from build123d import *

# Parameters (mm, degrees)
F1_DEPTH  = 20
F3_DEPTH  = 10
F4_R      = 1.25
F5_DEPTH  = 2.2
F7_DEPTH  = 10
F9_R      = 1.25
F10_DEPTH = 28.001
F11_R     = 2
F14_DEPTH = 1.5
F16_W     = 20
F16_H     = 10
F17_DEPTH = 26.7
F19_R     = 1.25
F20_DEPTH = 32.1
F22_W     = 20
F22_H     = 9.2705127583
F23_DEPTH = 6.9
F24_DEPTH = 2.9
F25_R     = 1.25
F26_DEPTH = 12.5


with BuildPart() as f1:
    # F0 (on Top) → F1 (new body)
    with BuildSketch(Plane.XY):
        with BuildLine():
            Line((-17.4218026286, 7.8075558554), (-19.6106751933, 7.8075558554))
            ThreePointArc((-19.6106751933, 7.8075558554), (-13.947676921, -0.1749805422), (-8.2846786486, 7.8075558554))
            Line((-8.2846786486, 7.8075558554), (-10.4735512133, 7.8075558554))
            ThreePointArc((-10.4735512133, 7.8075558554), (-13.947676921, 1.8250194578), (-17.4218026286, 7.8075558554))
        make_face()
    extrude(amount=F1_DEPTH)

    # F2 (on Top) → F3 (join, symmetric)
    with BuildSketch(Plane.XY):
        Polygon((-3.947676921, 1.8250194578), (-13.947676921, 1.8250194578), (-23.947676921, 1.8250194578), (-23.947676921, -1.1749805422), (-3.947676921, -1.1749805422), align=None)
    extrude(amount=F3_DEPTH, both=True)

    # F4 (on Front) → F5 (cut, symmetric)
    with BuildSketch(Plane.XZ):
        with Locations((-9.197676921, -6)):
            Circle(F4_R)
        with Locations((-18.697676921, -6)):
            Circle(F4_R)
    extrude(amount=F5_DEPTH, both=True, mode=Mode.SUBTRACT)

    # F6 (on face) → F7 (join, through all)
    with BuildSketch(Plane.XY.offset(10)):
        with BuildLine():
            Line((-3.947676921, 1.8250194578), (-9.475540966, 1.8250194578))
            ThreePointArc((-9.475540966, 1.8250194578), (-13.947676921, -0.1749805422), (-18.419812876, 1.8250194578))
            Line((-18.419812876, 1.8250194578), (-23.947676921, 1.8250194578))
            Line((-23.947676921, 1.8250194578), (-23.947676921, -1.1749805422))
            Line((-23.947676921, -1.1749805422), (-3.947676921, -1.1749805422))
            Line((-3.947676921, -1.1749805422), (-3.947676921, 1.8250194578))
        make_face()
    extrude(amount=F7_DEPTH)

    # F9 (on offset) → F10 (cut, through all)
    with BuildSketch(Plane(origin=(0, 26.8250194578, 0), x_dir=(-1, 0, 0), z_dir=(0, 1, 0))):
        with Locations((23.947676921, -6)):
            Circle(F9_R)
        with Locations((3.947676921, -6)):
            Circle(F9_R)
    extrude(amount=-F10_DEPTH, mode=Mode.SUBTRACT)

    # F11
    f11_edges = [f1.edges().sort_by_distance(p)[0] for p in [
        (-23.947677, 0.325019, -10),
        (-3.947677, 0.325019, -10),
    ]]
    fillet(f11_edges, radius=F11_R)

    # F13 (on offset) → F14 (join)
    with BuildSketch(Plane.XZ.offset(1.1749805422)):
        with BuildLine():
            ThreePointArc((-23.947676921, -4.75), (-22.697676921, -6), (-23.947676921, -7.25))
            Line((-23.947676921, -7.25), (-23.947676921, -8))
            ThreePointArc((-23.947676921, -8), (-23.3618904833, -9.4142135624), (-21.947676921, -10))
            Line((-21.947676921, -10), (-5.947676921, -10))
            ThreePointArc((-5.947676921, -10), (-4.5334633586, -9.4142135624), (-3.947676921, -8))
            Line((-3.947676921, -8), (-3.947676921, -7.25))
            ThreePointArc((-3.947676921, -7.25), (-5.197676921, -6), (-3.947676921, -4.75))
            Line((-3.947676921, -4.75), (-3.947676921, 20))
            Line((-3.947676921, 20), (-23.947676921, 20))
            Line((-23.947676921, 20), (-23.947676921, -4.75))
        make_face()
    extrude(amount=F14_DEPTH)

    # F16 (on offset) → F17 (cut)
    with BuildSketch(Plane(origin=(0, 26.8250194578, 0), x_dir=(-1, 0, 0), z_dir=(0, 1, 0))):
        with Locations((13.947676921, -5)):
            Rectangle(F16_W, F16_H)
    extrude(amount=-F17_DEPTH, mode=Mode.SUBTRACT)

    # F19 (on offset) → F20 (cut)
    with BuildSketch(Plane.XZ.offset(25)):
        with Locations((-9.197676921, -6)):
            Circle(F19_R)
        with Locations((-18.697676921, -6)):
            Circle(F19_R)
    extrude(amount=-F20_DEPTH, mode=Mode.SUBTRACT)

    # F22 (on offset) → F23 (cut)
    with BuildSketch(Plane.XY.offset(11.9)):
        with Locations((-13.947676921, 6.460275837)):
            Rectangle(F22_W, F22_H)
    extrude(amount=-F23_DEPTH, mode=Mode.SUBTRACT)

    # F22 (on offset) → F24 (cut)
    with BuildSketch(Plane.XY.offset(11.9)):
        with Locations((-13.947676921, 6.460275837)):
            Rectangle(F22_W, F22_H)
    extrude(amount=F24_DEPTH, mode=Mode.SUBTRACT)

    # F25 (on offset) → F26 (cut, symmetric)
    with BuildSketch(Plane(origin=(0, 1.8250194578, 0), x_dir=(-1, 0, 0), z_dir=(0, 1, 0))):
        with Locations((8.2846786486, 10.0688289385)):
            Circle(F25_R)
        with Locations((19.6106751933, 10.0688289385)):
            Circle(F25_R)
    extrude(amount=F26_DEPTH, both=True, mode=Mode.SUBTRACT)


solid = f1.part
Geometry check sheet. Reference: the model listing, model coordinates, mm. A direction names the side the tool comes from. Give positions to 0.01 mm unless a question says otherwise; leave off trailing zeros. Write each loop counter-clockwise with the first axis right and the second up, starting at its lowest first coordinate (ties: lowest second). Pieces come first, ordered by that corner, then holes. Notation, with made-up numbers: M -15,-4 L 40,-4 A18 ccw 40,23 Z; hole C 71.5,-6.75 d10. An arc over 180 degrees is marked long. Answer as CSV lines item,"result". Start each with the question number.
Q1. Section check B-B, the plane y = 3.25. Record the cut outline in (x, z), then the cut area to 3 significant figures.
Q2. Go/stop test with flat-tipped pins: pin 1 (5 mm diameter, centred on x = -18, y = 3.5, fed in from -Z); pin 2 (3 mm diameter, centred on x = -8.28, z = 10.07, fed in from +Y) (3 decimals). Record where each tip stops, or that it passes through.
Q3. Release check for a two-part mould opening along X. For faces 1 (the face through (-22.7, -1.26, -5.97)), 2 (the face through (-14, -1, -10)), 3 (the face through (-8.01, -0.39, 8.85)), 4 (the face through (-13.831, 1.827, 2.465)) record: pulls with the +X half, pulls with the -X half, needs draft (parallel to the pull), parting line crosses it, or undercut.
Q4. Section check A-A, the plane z = -6. Record the cut outline in (x, y).
Q5. Material ranges on L1, parallel to Z at x = -9.5, y = 4.75; L2, parallel to Y at x = -7.25, z = 6; L3, parallel to Y at x = -15.75, z = -3.75, recorded low to high.
Q6. Section check C-C, the plane z = 17.75. Record the cut outline in (x, y).
Q7. Section check D-D, the plane x = -19.25. Record the cut outline in (y, z).
Q8. Tool access check on faces 5 (the face through (-9, 7.808, 17)), 6 (the face through (-14, 1, 0)), 7 (the face through (-18.3, 4.9, 5)). Record the directions out of +Z, -Z, +X, -X, +Y, -Y that give a thin tool (end or side, any length) a straight path to the whole face; none if there is none.
Geometry says:
1,outline,"M -19.37,0 L -17.01,0 L -17.01,5 L -19.37,5 Z; M -19.37,14.8 L -17.01,14.8 L -17.01,20 L -19.37,20 Z; M -10.89,0 L -8.53,0 L -8.53,5 L -10.89,5 Z; M -10.89,14.8 L -8.53,14.8 L -8.53,20 L -10.89,20 Z"
1,area,"48.1 mm^2"
2,pin 1,"z = 0"
2,pin 2,"y = 1.825"
3,face 1,"pulls with the -X half"
3,face 2,"needs draft"
3,face 3,"undercut"
3,face 4,"undercut"
4,outline,"M -22.7,-2.67 L -19.95,-2.67 L -19.95,0.13 L -22.7,0.13 Z; M -17.45,-2.67 L -10.45,-2.67 L -10.45,0.13 L -17.45,0.13 Z; M -7.95,-2.67 L -5.2,-2.67 L -5.2,0.13 L -7.95,0.13 Z"
5,L1,"0 to 5, 14.8 to 20"
5,L2,"-2.67 to 1.83"
5,L3,"-2.67 to 0.13"
6,outline,"M -23.95,-2.67 L -3.95,-2.67 L -3.95,1.83 L -9.48,1.83 A6 ccw -8.28,7.81 L -10.47,7.81 A4 cw long -17.42,7.81 L -19.61,7.81 A6 ccw -18.42,1.83 L -23.95,1.83 Z"
7,outline,"M -2.67,-10 L 0.13,-10 L 0.13,-7.12 L -2.67,-7.12 Z; M -2.67,-4.88 L 0.13,-4.88 L 0.13,0 L 1.83,0 L 1.83,8.87 L -2.67,8.87 Z; M -2.67,11.27 L 1.83,11.27 L 1.83,20 L -2.67,20 Z; M 3.02,0 L 7.81,0 L 7.81,5 L 3.02,5 Z; M 3.02,14.8 L 7.81,14.8 L 7.81,20 L 3.02,20 Z"
8,face 5,"+Z, -Z, +X, -X, +Y"
8,face 6,"-Z, +X, -X, +Y"
8,face 7,"+X, -X, +Y"
